Input: part model. Units: mm. Frame: model coordinates. Face numbers are marked on the shaded views. A direction names the side the tool comes from. Coordinates: 2 decimals unless noted, no trailing zeros. Order: outer loops, then holes, each group sorted by start corner. A loop starts at its lowest first (then second) coordinate and runs counter-clockwise, first axis right, second up.
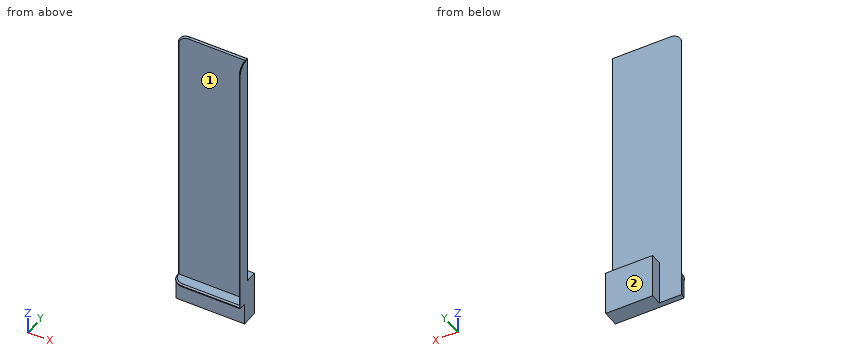
from build123d import *

# Parameters (mm, degrees)
F0_W      = 76.2
F0_H      = 304.8
F1_DEPTH  = 1.778
F2_W      = 76.2
F2_H      = 2.54
F3_DEPTH  = 12.7
F4_W      = 14.478
F4_H      = 304.8
F5_DEPTH  = 1.778
F4_W_2    = 0.1264255261
F4_H_2    = 0.0905882334
F6_W      = 77.978
F6_H      = 5.842
F7_DEPTH  = 25.4
F8_W      = 52.324
F8_H      = 50.8
F9_DEPTH  = 10.16
F11_W     = 52.832
F11_H     = 50.8
F12_DEPTH = 12.7
F13_R     = 12.7
F14_R     = 12.7
F15_R     = 12.7
F16_SIZE  = 1.524
F17_SIZE  = 1.523


# Not quite as in the source:
# - a fillet or chamfer is up to 0.001 mm smaller than in the source, because OpenCascade refuses the exact size


with BuildPart() as f1:
    # F0 (on Front) → F1 (new body)
    with BuildSketch(Plane.XZ):
        with Locations((38.1, 152.4)):
            Rectangle(F0_W, F0_H)
    extrude(amount=F1_DEPTH)

    # F2 (on face) → F3 (join)
    with BuildSketch(Plane.XZ.offset(1.778)):
        with Locations((38.1, 1.27)):
            Rectangle(F2_W, F2_H)
    extrude(amount=F3_DEPTH)

    # F4 (on face) → F5 (join)
    with BuildSketch(Plane.YZ.offset(76.2)):
        with Locations((-7.239, 152.4)):
            Rectangle(F4_W, F4_H)
    extrude(amount=F5_DEPTH)

    # F6 (on face) → F7 (join)
    with BuildSketch(Plane(origin=(0, 0, 0), x_dir=(1, 0, 0), z_dir=(0, 0, -1))):
        with Locations((38.989, 2.921)):
            Rectangle(F6_W, F6_H)
    extrude(amount=F7_DEPTH)

    # F11 (on face) → F12 (join)
    with BuildSketch(Plane(origin=(0, 0, 0), x_dir=(-1, 0, 0), z_dir=(0, 1, 0))):
        with Locations((-51.562, 0)):
            Rectangle(F11_W, F11_H)
    extrude(amount=F12_DEPTH)

    # F13
    f13_edges = [f1.edges().sort_by_distance(p)[0] for p in [
        (0, -0.889, 304.8),
    ]]
    fillet(f13_edges, radius=F13_R)

    # F14
    f14_edges = [f1.edges().sort_by_distance(p)[0] for p in [
        (77.089, -14.478, 304.8),
    ]]
    fillet(f14_edges, radius=F14_R)

    # F15
    f15_edges = [f1.edges().sort_by_distance(p)[0] for p in [
        (0, -14.478, 1.27),
    ]]
    fillet(f15_edges, radius=F15_R)

    # F16
    f16_edges = [f1.edges().sort_by_distance(p)[0] for p in [
        (0, -1.778, 147.32),
    ]]
    chamfer(f16_edges, length=F16_SIZE)

    # F17 (size 1.524 in the source; OpenCascade refuses exactly that, so slightly less here)
    f17_edges = [f1.edges().sort_by_distance(p)[0] for p in [
        (3.719744, -10.758256, 2.54),
        (44.45, -14.478, 2.54),
        (76.2, -14.478, 147.32),
    ]]
    chamfer(f17_edges, length=F17_SIZE)


with BuildPart() as f5:
    # F4 (on face) → F5, piece 2 (new body)
    with BuildSketch(Plane.YZ.offset(76.2)):
        with Locations((1.1594051612, 0.5721470225)):
            Rectangle(F4_W_2, F4_H_2)
    extrude(amount=F5_DEPTH)


with BuildPart() as f9:
    # F8 (on face) → F9 (new body)
    with BuildSketch(Plane(origin=(0, 0, 0), x_dir=(-1, 0, 0), z_dir=(0, 1, 0))):
        with Locations((-51.816, 0)):
            Rectangle(F8_W, F8_H)
    extrude(amount=F9_DEPTH)


solid = f1.part
Item 1: Pin query (flat end, axial travel): pin 1 Ø12.5 at (x, z) = (34.5, -9) entering from -Y; pin 2 Ø10 at (y, z) = (-10, 169) entering from -X; pin 3 Ø2.5 at (x, y) = (54.5, -9.5) entering from -Z. Return the tip coordinate at first contact, or that it passes through.
Response values:
pin 1: stops at y = -5.84
pin 2: stops at x = 76.2
pin 3: stops at z = 0
Item 2: Cut plane A-A on x = 16.5. Return loops of the section in (y, z) (3 decimals).
Response values:
outline: (-14.478, 0) - (-5.842, 0) - (-5.842, -25.4) - (0, -25.4) - (0, 304.8) - (-0.254, 304.8) - (-1.778, 303.276) - (-1.778, 2.54) - (-12.955, 2.54) - (-14.478, 1.017) - close
Item 3: Ray query, probe 1 along Y at (x, z) = (40, -9); probe 2 along Y at (x, z) = (8, 162.5); probe 3 along Z at (x, y) = (19, -3.5). Return the intervals inside material, ascending.
Response values:
probe 1: y = -5.84 to 12.7
probe 2: y = -1.78 to 0
probe 3: z = -25.4 to 2.54
Item 4: Cut plane C-C on x = 40.5. Return loops of the section in (y, z) (3 decimals), then the cut area to 3 significant figures.
Response values:
outline: (-14.478, 0) - (-5.842, 0) - (-5.842, -25.4) - (12.7, -25.4) - (12.7, 25.4) - (0, 25.4) - (0, 304.8) - (-0.254, 304.8) - (-1.778, 303.276) - (-1.778, 2.54) - (-12.955, 2.54) - (-14.478, 1.017) - close
area: 1,370 mm2
Item 5: Cut plane B-B on z = 93. Return loops of the section in (x, y) (3 decimals), then the cut area to 3 significant figures.
Response values:
outline: (0, -0.254) - (1.524, -1.778) - (76.2, -1.778) - (76.2, -12.955) - (77.723, -14.478) - (77.978, -14.478) - (77.978, 0) - (0, 0) - close
area: 159 mm2
Item 6: Access query for the marked faces 1 and 2. Directions: +Z, -Z, +X, -X, +Y, -Y. A direction counts if a zero-diameter tool reaches every point of the face in a straight line with its end or side. Return the directions, or none.
Response values:
face 1: +Z, -X, -Y
face 2: +Z, -Z, +X, -X, +Y
